from build123d import *

# Parameters (mm, degrees)
ESBO_O1_W                = 80
ESBO_O1_H                = 80
RESSALTO_EXTRUS_O1_DEPTH = 15
ESBO_O2_W                = 42.2
ESBO_O2_H                = 42.2
CORTE_EXTRUS_O1_DEPTH    = 13
FILETE1_R                = 5
ESBO_O3_R                = 11.1
ESBO_O3_R_2              = 2
CORTE_EXTRUS_O2_DEPTH    = 3
ESBO_O4_R                = 7.7
CORTE_EXTRUS_O3_DEPTH    = 16
FILETE2_R                = 5


with BuildPart() as part:
    # Esboço1 → Ressalto-extrusão1 (new body)
    with BuildSketch(Plane(origin=(0, 0, 0), x_dir=(1, 0, 0), z_dir=(0, 1, 0))):
        Rectangle(ESBO_O1_W, ESBO_O1_H)
    extrude(amount=RESSALTO_EXTRUS_O1_DEPTH)

    # Esboço2 → Corte-extrusão1 (cut)
    with BuildSketch(Plane(origin=(0, 15, 0), x_dir=(1, 0, 0), z_dir=(0, 1, 0))):
        Rectangle(ESBO_O2_W, ESBO_O2_H)
    extrude(amount=-CORTE_EXTRUS_O1_DEPTH, mode=Mode.SUBTRACT)

    # Filete1
    filete1_edges = [part.edges().sort_by_distance(p)[0] for p in [
        (-21.1, 8.5, 21.1),
        (-21.1, 8.5, -21.1),
        (21.1, 8.5, -21.1),
        (21.1, 8.5, 21.1),
    ]]
    fillet(filete1_edges, radius=FILETE1_R)

    # Esboço3 → Corte-extrusão2 (cut, through all)
    with BuildSketch(Plane(origin=(0, 2, 0), x_dir=(1, 0, 0), z_dir=(0, 1, 0))):
        Circle(ESBO_O3_R)
        with Locations((-15.5, 15.5)):
            Circle(ESBO_O3_R_2)
        with Locations((15.5, 15.5)):
            Circle(ESBO_O3_R_2)
        with Locations((15.5, -15.5)):
            Circle(ESBO_O3_R_2)
        with Locations((-15.5, -15.5)):
            Circle(ESBO_O3_R_2)
    extrude(amount=-CORTE_EXTRUS_O2_DEPTH, mode=Mode.SUBTRACT)

    # Esboço4 → Corte-extrusão3 (cut, through all)
    with BuildSketch(Plane(origin=(0, 15, 0), x_dir=(1, 0, 0), z_dir=(0, 1, 0))):
        with Locations((-30, 30)):
            Circle(ESBO_O4_R)
        with Locations((30, 30)):
            Circle(ESBO_O4_R)
        with Locations((30, -30)):
            Circle(ESBO_O4_R)
        with Locations((-30, -30)):
            Circle(ESBO_O4_R)
    extrude(amount=-CORTE_EXTRUS_O3_DEPTH, mode=Mode.SUBTRACT)

    # Filete2
    filete2_edges = [part.edges().sort_by_distance(p)[0] for p in [
        (-40, 7.5, -40),
        (40, 7.5, -40),
        (40, 7.5, 40),
        (-40, 7.5, 40),
    ]]
    fillet(filete2_edges, radius=FILETE2_R)


solid = part.part
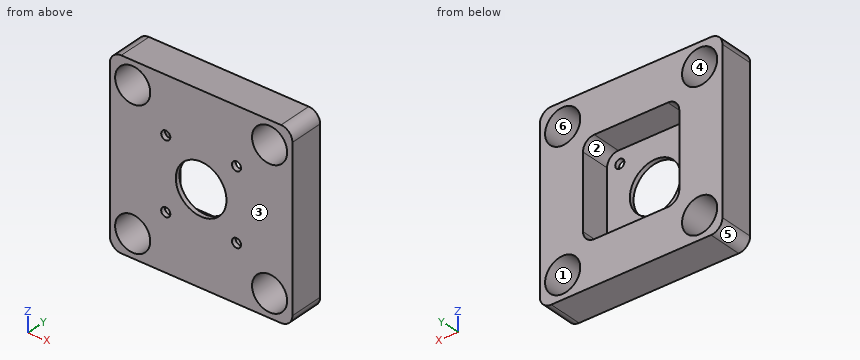
Could you check a few things on this model? Use its own coordinates, in mm. Face numbers are marked on the shaded views. A direction names the side the tool comes from. Coordinates: 2 decimals unless noted, no trailing zeros. Write each loop counter-clockwise with the first axis right and the second up, starting at its lowest first coordinate (ties: lowest second). Pieces come first, ordered by that corner, then holes. Notation, with made-up numbers: M 25,-5 L 38,-5 A22 ccw 38,30 Z; hole C 32,-8 d7. An arc over 180 degrees is marked long. One line per question, with ' | ' between items.
1) For the marked faces 1 and 2, which set-ups out of +Z, -Z, +X, -X, +Y, -Y let a thin tool reach every point of the face, with its end or its side?
Checks:
face 1: +Y, -Y | face 2: +Y
2) I need wall thicknesses on probe 1 along Z at (x, y) = (30, 3.75); probe 2 along X at (y, z) = (1.15, 15.5). Which ranges of each line are inside material? Lowest first, please. Write a range as [from, to].
Checks:
probe 1: [-40, -37.7], [-22.3, 22.3], [37.7, 40] | probe 2: [-40, -17.5], [-13.5, 13.5], [17.5, 40]
3) Imagine slicing it at A-A, the plane z = -30. Write out the boundary of the cut face in (x, y).
Checks:
outline: M -40,0 L -37.7,0 L -37.7,15 L -40,15 Z; M -22.3,0 L 22.3,0 L 22.3,15 L -22.3,15 Z; M 37.7,0 L 40,0 L 40,15 L 37.7,15 Z
4) For pin 1 Ø4 at (x, z) = (10.5, 13) entering from -Y; pin 2 Ø5 at (x, z) = (-15.5, -15.5) entering from +Y; pin 3 Ø14 at (x, z) = (30, 30) entering from +Y, each with a flat end and sliding along its axis, tell me the tip position at first contact or that it passes through.
Checks:
pin 1: y = 0 | pin 2: y = 2 | pin 3: through
5) Imagine slicing it at D-D, the plane y = 4. Write out the boundary of the cut face in (x, z).
Checks:
outline: M -40,-35 A5 ccw -35,-40 L 35,-40 A5 ccw 40,-35 L 40,35 A5 ccw 35,40 L -35,40 A5 ccw -40,35 Z; hole C -30,-30 d15.4; hole C -30,30 d15.4; hole M -21.1,-16.1 A5 ccw -16.1,-21.1 L 16.1,-21.1 A5 ccw 21.1,-16.1 L 21.1,16.1 A5 ccw 16.1,21.1 L -16.1,21.1 A5 ccw -21.1,16.1 Z; hole C 30,-30 d15.4; hole C 30,30 d15.4
6) If we mould it in two halves opening along Z, with no side actions, what happens to the marked faces 3, 4, 5 and 6? For each: released by +Z, released by -Z, zero draft, split by the parting line, or undercut.
Checks:
face 3: zero draft | face 4: undercut | face 5: released by -Z | face 6: undercut
7) Imagine slicing it at C-C, the plane x = 0. Write out the boundary of the cut face in (y, z).
Checks:
outline: M 0,-40 L 15,-40 L 15,-21.1 L 2,-21.1 L 2,-11.1 L 0,-11.1 Z; M 0,11.1 L 2,11.1 L 2,21.1 L 15,21.1 L 15,40 L 0,40 Z
8) Imagine slicing it at B-B, the plane x = 30. Write out the boundary of the cut face in (y, z), and give its area (3 significant figures).
Checks:
outline: M 0,-40 L 15,-40 L 15,-37.7 L 0,-37.7 Z; M 0,-22.3 L 15,-22.3 L 15,22.3 L 0,22.3 Z; M 0,37.7 L 15,37.7 L 15,40 L 0,40 Z | area: 738 mm²
